from build123d import *

# Parameters (mm, degrees)
F0_W           = 75
F0_H           = 60
F1_DEPTH       = 6
F2_W           = 75
F2_H           = 6
F3_DEPTH       = 24
F5_D           = 3
F5_CBORE_D     = 6
F5_CBORE_DEPTH = 3.5
F4_R           = 11
F6_DEPTH       = 6.001
F4_R_2         = 2
F7_DEPTH       = 6.001
F9_D           = 8
F9_CBORE_D     = 13
F9_CBORE_DEPTH = 4
F10_W          = 3.5
F10_H          = 10
F11_DEPTH      = 60.001
F12_SIZE       = 0.8
F13_R          = 2


with BuildPart() as f1:
    # F0 (on Top) → F1 (new body)
    with BuildSketch(Plane.XY):
        Rectangle(F0_W, F0_H)
    extrude(amount=F1_DEPTH)

    # F2 (on face) → F3 (join)
    with BuildSketch(Plane.XY.offset(6)):
        with Locations((0, 27)):
            Rectangle(F2_W, F2_H)
    extrude(amount=F3_DEPTH)

    # F5 (through all)
    with Locations(Plane.XY.offset(6)):
        with Locations((-23, 15), (8, 15), (8, -16), (-23, -16)):
            CounterBoreHole(F5_D / 2, F5_CBORE_D / 2, F5_CBORE_DEPTH)

    # F4 (on face) → F6 (cut, through all)
    with BuildSketch(Plane.XY.offset(6)):
        with Locations((-7.5, -0.5)):
            Circle(F4_R)
    extrude(amount=-F6_DEPTH, mode=Mode.SUBTRACT)

    # F4 (on face) → F7 (cut, through all)
    with BuildSketch(Plane.XY.offset(6)):
        with Locations((-29, -10)):
            Circle(F4_R_2)
        with Locations((14, -10)):
            Circle(F4_R_2)
    extrude(amount=-F7_DEPTH, mode=Mode.SUBTRACT)

    # F9 (through all)
    with Locations(Plane.XZ.offset(-24)):
        with Locations((-22.5, 15), (7.5, 15)):
            CounterBoreHole(F9_D / 2, F9_CBORE_D / 2, F9_CBORE_DEPTH)

    # F10 (on face) → F11 (cut, through all)
    with BuildSketch(Plane(origin=(0, 30, 0), x_dir=(-1, 0, 0), z_dir=(0, 1, 0))):
        with Locations((35.75, 15)):
            Rectangle(F10_W, F10_H)
    extrude(amount=-F11_DEPTH, mode=Mode.SUBTRACT)

    # F12
    f12_edges = [f1.edges().sort_by_distance(p)[0] for p in [
        (-37.5, 27, 20),
        (-37.5, 27, 10),
    ]]
    chamfer(f12_edges, length=F12_SIZE)

    # F13
    f13_edges = [f1.edges().sort_by_distance(p)[0] for p in [
        (-37.5, 27, 30),
    ]]
    fillet(f13_edges, radius=F13_R)


solid = f1.part
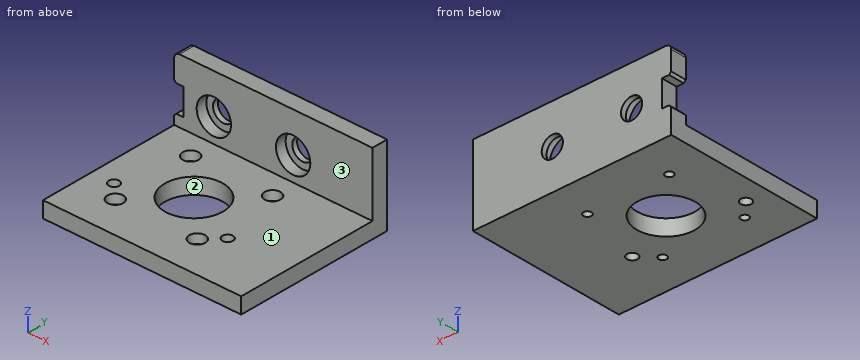
Check sheet for the modelled part. Datum: model origin and axes. Units: mm. Face numbers are marked on the shaded views. Round coordinates to 2 decimals unless told otherwise and drop trailing zeros. Order: outer loops, then holes, each group sorted by start corner. A loop starts at its lowest first (then second) coordinate and runs counter-clockwise, first axis right, second up.
(1) Cross-section at C-C, the plane y = 15. Enter the section's corners in (x, z).
(2) Scan lines: probe 1 along Y at (x, z) = (8, 4.6); probe 2 along X at (y, z) = (25, 18.75); probe 3 along Z at (x, y) = (18, -9). Record each from-to range of solid material in increasing order.
(3) Draft check along Y on the marked faces 1, 2 and 3. Enter one of: pulls with the +Y half, pulls with the -Y half, needs draft (parallel to the pull), parting line crosses it, or undercut.
(4) Go/stop test with flat-tipped pins: P1, Ø3.5, axis at x = 8, y = -16, coming from the +Z side; P2, Ø6.5, axis at x = 9.5, y = 14, coming from the +Z side; P3, Ø8, axis at x = -19, z = 27, coming from the -Y side. Record where each tip stops, or that it passes through.
(5) Cross-section at D-D, the plane x = -12. Enter the section's corners in (y, z), and give its area (3 significant figures).
(6) Cross-section at B-B, the plane z = 15. Enter the section's corners in (x, y).
(7) Cross-section at A-A, the plane y = -0.5. Enter the section's corners in (x, z), and give its area (3 significant figures).
Check sheet entries:
1. outline: (-37.5, 0) - (-24.5, 0) - (-24.5, 2.5) - (-26, 2.5) - (-26, 6) - (-37.5, 6) - close; (-21.5, 0) - (6.5, 0) - (6.5, 2.5) - (5, 2.5) - (5, 6) - (-20, 6) - (-20, 2.5) - (-21.5, 2.5) - close; (9.5, 0) - (37.5, 0) - (37.5, 6) - (11, 6) - (11, 2.5) - (9.5, 2.5) - close
2. probe 1: y = -30 to -19, -13 to 12, 18 to 30
2. probe 2: x = -34 to -27.81, -17.19 to 2.19, 12.81 to 37.5
2. probe 3: z = 0 to 6
3. face 1: needs draft
3. face 2: undercut
3. face 3: pulls with the -Y half
4. P1: stops at z = 2.5
4. P2: stops at z = 6
4. P3: stops at y = 24
5. outline: (-30, 0) - (-10.54, 0) - (-10.54, 6) - (-30, 6) - close; (9.54, 0) - (30, 0) - (30, 30) - (24, 30) - (24, 6) - (9.54, 6) - close
5. area: 384 mm2
6. outline: (-34, 24) - (-29, 24) - (-29, 28) - (-26.5, 28) - (-26.5, 30) - (-34, 30) - close; (-18.5, 28) - (-16, 28) - (-16, 24) - (1, 24) - (1, 28) - (3.5, 28) - (3.5, 30) - (-18.5, 30) - close; (11.5, 28) - (14, 28) - (14, 24) - (37.5, 24) - (37.5, 30) - (11.5, 30) - close
7. outline: (-37.5, 0) - (-18.5, 0) - (-18.5, 6) - (-37.5, 6) - close; (3.5, 0) - (37.5, 0) - (37.5, 6) - (3.5, 6) - close
7. area: 318 mm2
